from build123d import *

# Parameters (mm, degrees)
SKETCH2_R          = 3
CUT_EXTRUDE1_DEPTH = 10
CIRPATTERN1_COUNT  = 6
SKETCH3_R          = 10
CUT_EXTRUDE2_DEPTH = 10


with BuildPart() as part:
    # Sketch1 → Revolve1 (revolve)
    with BuildSketch(Plane.XY):
        Polygon((0, 35), (5, 35), (5, 21), (8, 21), (8, 16), (5, 16), (5, 0), (0, 0), align=None)
    revolve(axis=Axis((5, 0, 0), (-1, 0, 0)))

    # Sketch2 → Cut-Extrude1 (cut)
    with BuildSketch(Plane(origin=(5, 0, 0), x_dir=(0, 0, -1), z_dir=(1, 0, 0))):
        with Locations((27.5, 0)):
            Circle(SKETCH2_R)
    cut_extrude1 = extrude(amount=-CUT_EXTRUDE1_DEPTH, mode=Mode.SUBTRACT)

    # CirPattern1: Cut-Extrude1 ×6 about axis
    cirpattern1_axis = Axis((0, 0, 0), (1, 0, 0))
    for i in range(1, CIRPATTERN1_COUNT):
        add(cut_extrude1.rotate(cirpattern1_axis, i * 360 / CIRPATTERN1_COUNT), mode=Mode.SUBTRACT)

    # Sketch3 → Cut-Extrude2 (cut)
    with BuildSketch(Plane(origin=(5, 0, 0), x_dir=(0, 0, -1), z_dir=(1, 0, 0))):
        Circle(SKETCH3_R)
    extrude(amount=-CUT_EXTRUDE2_DEPTH, mode=Mode.SUBTRACT)


solid = part.part
Check sheet for the modelled part. Datum: model origin and axes. Units: mm. A direction names the side the tool comes from. Give positions to 0.01 mm unless a question says otherwise; leave off trailing zeros. Order: outer loops, then holes, each group sorted by start corner. A loop starts at its lowest first (then second) coordinate and runs counter-clockwise, first axis right, second up. Notation, with made-up numbers: (36.5, 55) - (72.5, 55) arc R16 cw to (72.5, 84) - close; hole circle Ø2 at (3, -1). An arc over 180 degrees is marked (long way). Answer as CSV lines item,"result".
1. Section check D-D (y = 19). Record the boundary of the cut face in (x, z), then the cut area to 3 significant figures.
Result sheet:
outline,"(0, -29.39) - (5, -29.39) - (5, -8.94) - (8, -8.94) - (8, 8.94) - (5, 8.94) - (5, 29.39) - (0, 29.39) - close"
area,"348 mm²"
2. Section check A-A (z = 0). Record the boundary of the cut face in (x, y), then the cut area to 3 significant figures.
Result sheet:
outline,"(0, -35) - (5, -35) - (5, -21) - (8, -21) - (8, -16) - (5, -16) - (5, -10) - (0, -10) - close; (0, 10) - (5, 10) - (5, 16) - (8, 16) - (8, 21) - (5, 21) - (5, 35) - (0, 35) - close"
area,"280 mm²"
3. Go/stop test with flat-tipped pins: P1, Ø23, axis at y = 0, z = 0, coming from the +X side; P2, Ø2, axis at x = 5, z = -18, coming from the -Y side; P3, Ø2, axis at x = 5.5, z = -28, coming from the +Y side. Record where each tip stops, or that it passes through.
Result sheet:
P1,"x = 5"
P2,"y = -30.59"
P3,"y = 22.11"
4. Section check B-B (y = 0). Record the boundary of the cut face in (x, z), then the cut area to 3 significant figures.
Result sheet:
outline,"(0, -35) - (5, -35) - (5, -30.5) - (0, -30.5) - close; (0, -24.5) - (5, -24.5) - (5, -21) - (8, -21) - (8, -16) - (5, -16) - (5, -10) - (0, -10) - close; (0, 10) - (5, 10) - (5, 16) - (8, 16) - (8, 21) - (5, 21) - (5, 24.5) - (0, 24.5) - close; (0, 30.5) - (5, 30.5) - (5, 35) - (0, 35) - close"
area,"220 mm²"
5. Tool access check on faces 1 (the face through (6.48, -3.47, 15.62)), 2 (the face through (2.5, 0.1, -24.5)). Record the directions out of +Z, -Z, +X, -X, +Y, -Y that give a thin tool (end or side, any length) a straight path to the whole face; none if there is none.
Result sheet:
face 1,"+X"
face 2,"+X, -X"
6. Mould release check, pull along Z, two halves, no side actions. Record for faces 3 (the face through (2.54, -26.79, -14.14)), 4 (the face through (6.52, 20.03, -6.31)), 5 (the face through (5, 15, 15)): released by +Z, released by -Z, zero draft, split by the parting line, or undercut.
Result sheet:
face 3,"undercut"
face 4,"split by the parting line"
face 5,"zero draft"
7. Section check C-C (x = 6.75). Record the boundary of the cut face in (y, z), then the cut area to 3 significant figures.
Result sheet:
outline,"circle Ø42 at (0, 0); hole circle Ø32 at (0, 0)"
area,"581 mm²"
8. Scan lines: probe 1 along Z at (x, y) = (6, 0); probe 2 along Z at (x, y) = (3.25, 2.5); probe 3 along Y at (x, z) = (3.85, 0). Record each from-to range of solid material in increasing order. Write a range as from..to.
Result sheet:
probe 1,"-21..-16, 16..21"
probe 2,"-34.91..-29.16, -25.84..-9.68, 9.68..25.84, 29.16..34.91"
probe 3,"-35..-10, 10..35"
